Model file for the job. Use its own axes, mm. A direction names the side the tool comes from. Round coordinates to 2 decimals unless told otherwise and drop trailing zeros. Order: outer loops, then holes, each group sorted by start corner. A loop starts at its lowest first (then second) coordinate and runs counter-clockwise, first axis right, second up. Notation, with made-up numbers: (-31, 21.5) -> (-18, 21.5) arc R27 cw to (-18, 54.5) -> close; hole circle Ø2 at (-32, 88.25). An arc over 180 degrees is marked (long way). Use CSV: the item, a comma, the result in double quotes.
```python
from build123d import *

# Parameters (mm, degrees)
F0_W     = 240
F0_H     = 240
F1_DEPTH = 25
F2_W     = 10
F2_H     = 10
F2_H_2   = 200
F2_W_2   = 200
F3_DEPTH = 8


with BuildPart() as f1:
    # F0 (on Top) → F1 (new body)
    with BuildSketch(Plane.XY):
        Rectangle(F0_W, F0_H)
    extrude(amount=-F1_DEPTH)

    # F2 (on face) → F3 (cut)
    with BuildSketch(Plane.XY):
        with Locations((-105, 115)):
            Rectangle(F2_W, F2_H)
        with Locations((-105, 105)):
            Rectangle(F2_W, F2_H)
        with Locations((-115, 105)):
            Rectangle(F2_W, F2_H)
        with Locations((-105, 0)):
            Rectangle(F2_W, F2_H_2)
        with Locations((0, 105)):
            Rectangle(F2_W_2, F2_H)
        with Locations((105, 115)):
            Rectangle(F2_W, F2_H)
        with Locations((115, 105)):
            Rectangle(F2_W, F2_H)
        with Locations((105, 105)):
            Rectangle(F2_W, F2_H)
        with Locations((105, 0)):
            Rectangle(F2_W, F2_H_2)
        with Locations((105, -115)):
            Rectangle(F2_W, F2_H)
        with Locations((105, -105)):
            Rectangle(F2_W, F2_H)
        with Locations((115, -105)):
            Rectangle(F2_W, F2_H)
        with Locations((0, -105)):
            Rectangle(F2_W_2, F2_H)
        with Locations((-105, -105)):
            Rectangle(F2_W, F2_H)
        with Locations((-105, -115)):
            Rectangle(F2_W, F2_H)
        with Locations((-115, -105)):
            Rectangle(F2_W, F2_H)
    extrude(amount=-F3_DEPTH, mode=Mode.SUBTRACT)


solid = f1.part
```
Q1. Which spindle directions (+Z, -Z, +X, -X, +Y, -Y) get a long thin tool onto all of the face, cutting with end or side? Do faces 3 (the flat face through (-1, -115, 0)), 4 (the flat face through (115, -110, -4)), 5 (the flat face through (100, 1, -4)). Say none if no direction does.
From the geometry:
face 3,"+Z, +X, -X, +Y, -Y"
face 4,"+Z, +X, -X"
face 5,"+Z, +Y, -Y"
Q2. Cut at A-A (x = -71.5). Give the cut face in (y, z), plus the area to 3 significant figures.
From the geometry:
outline,"(-120, -25) -> (120, -25) -> (120, 0) -> (110, 0) -> (110, -8) -> (100, -8) -> (100, 0) -> (-100, 0) -> (-100, -8) -> (-110, -8) -> (-110, 0) -> (-120, 0) -> close"
area,"5,840 mm²"
Q3. Probe line 1 along X through (y, z) = (99.5, -4.5); line 2 along Z through (x, y) = (-100.5, -101.5). List the from-to ranges inside material, lowest first.
From the geometry:
line 1,"x = -120 to -110, -100 to 100, 110 to 120"
line 2,"z = -25 to -8"
Q4. Mould opens along X. For faces 1 (the flat face through (-110, 115, -4)), 2 (the flat face through (-115, 1, 0)) say: +X half, -X half, draft (parallel to the pull), parting line (faces both ways), or undercut.
From the geometry:
face 1,"undercut"
face 2,"draft"
